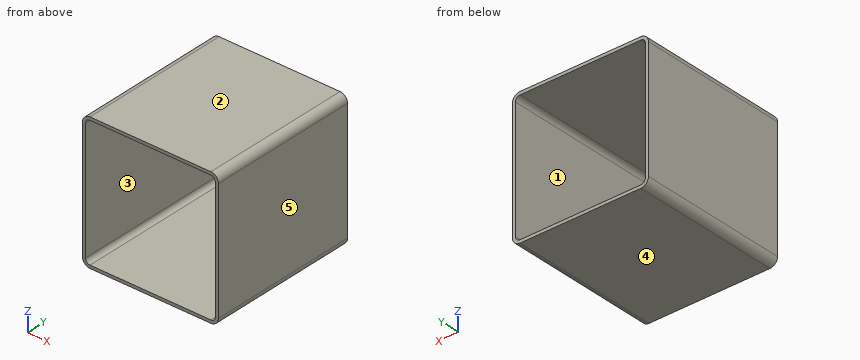
```python
from build123d import *

# Parameters (mm, degrees)
F0_W     = 90
F0_H     = 90
F0_W_2   = 86
F0_H_2   = 86
F1_DEPTH = 100
F2_R     = 5
F3_R     = 3


with BuildPart() as f1:
    # F0 (on Front) → F1 (new body)
    with BuildSketch(Plane.XZ):
        Rectangle(F0_W, F0_H)
        Rectangle(F0_W_2, F0_H_2, mode=Mode.SUBTRACT)
    extrude(amount=F1_DEPTH)

    # F2
    f2_edges = [f1.edges().sort_by_distance(p)[0] for p in [
        (45, -50, 45),
        (-45, -50, 45),
        (45, -50, -45),
        (-45, -50, -45),
    ]]
    fillet(f2_edges, radius=F2_R)

    # F3
    f3_edges = [f1.edges().sort_by_distance(p)[0] for p in [
        (-43, -50, 43),
        (43, -50, 43),
        (-43, -50, -43),
        (43, -50, -43),
    ]]
    fillet(f3_edges, radius=F3_R)


solid = f1.part
```
Here's how the part is built. I have some questions about the finished solid (model axes, mm). Face numbers are marked on the shaded views. A direction names the side the tool comes from. Round coordinates to 2 decimals unless told otherwise and drop trailing zeros. Order: outer loops, then holes, each group sorted by start corner. A loop starts at its lowest first (then second) coordinate and runs counter-clockwise, first axis right, second up. Notation, with made-up numbers: (27, 42) -> (48, 42) arc R15 ccw to (48, 63) -> close; hole circle Ø3 at (5, 80.5). An arc over 180 degrees is marked (long way). Use a Markdown table: item, result. Add a question column.
(1) Suppose I cut it at B-B, the plane x = -31. Please give me the cut outline in (y, z).
(2) Suppose I cut it at C-C, the plane y = -48. Please give me the cut outline in (x, z), and give its area (3 significant figures).
(3) If we mould it in two halves opening along Z, with no side actions, what happens to the marked faces 3, 4 and 5? For each: released by +Z, released by -Z, zero draft, split by the parting line, or undercut.
(4) I need wall thicknesses on line 1 along X through (y, z) = (-43, -27). Which ranges of the line are inside material? Lowest first, please.
(5) For the marked faces 1 and 2, which set-ups out of +Z, -Z, +X, -X, +Y, -Y let a thin tool reach every point of the face, with its end or its side?
(6) Suppose I cut it at A-A, the plane z = 10.5. Please give me the cut outline in (x, y), and give its area (3 significant figures).
Verdict:
| question | item | result |
|---|---|---|
| 1 | outline | (-100, -45) -> (0, -45) -> (0, -43) -> (-100, -43) -> close; (-100, 43) -> (0, 43) -> (0, 45) -> (-100, 45) -> close |
| 2 | outline | (-45, -40) arc R5 ccw to (-40, -45) -> (40, -45) arc R5 ccw to (45, -40) -> (45, 40) arc R5 ccw to (40, 45) -> (-40, 45) arc R5 ccw to (-45, 40) -> close; hole (-43, -40) arc R3 ccw to (-40, -43) -> (40, -43) arc R3 ccw to (43, -40) -> (43, 40) arc R3 ccw to (40, 43) -> (-40, 43) arc R3 ccw to (-43, 40) -> close |
| 2 | area | 690 mm2 |
| 3 | face 3 | undercut |
| 3 | face 4 | released by -Z |
| 3 | face 5 | zero draft |
| 4 | line 1 | -45 to -43, 43 to 45 |
| 5 | face 1 | +Y, -Y |
| 5 | face 2 | +Z, +X, -X, +Y, -Y |
| 6 | outline | (-45, -100) -> (-43, -100) -> (-43, 0) -> (-45, 0) -> close; (43, -100) -> (45, -100) -> (45, 0) -> (43, 0) -> close |
| 6 | area | 400 mm2 |
